Part print with two shaded views. Sizes in mm from the minimum x, y, z corner. Coordinates: 2 decimals unless noted, no trailing zeros. Write each loop counter-clockwise with the first axis right and the second up, starting at its lowest first coordinate (ties: lowest second). Pieces come first, ordered by that corner, then holes. Notation, with made-up numbers: M 78,32.25 L 95,32.25 A25 ccw 95,69.25 Z; hole C -25.5,40.25 d1. An arc over 180 degrees is marked long. One line per question, with ' | ' between items. Start each with the question number.
(1) Wall check: probe 1 along Z at (x, y) = (8, 0.95); probe 2 along X at (y, z) = (0.7, 5.25); probe 3 along Z at (x, y) = (9.25, 0.8). Give the ranges that are in metal, low to high.
(2) Cut at D-D (x = 2). Write the cut outline in (y, z).
(3) Cut at C-C (y = 0.85). Count the separate pieces of the cut face and the enclosed holes in it.
(4) Cut at A-A (z = 1.5). Write the cut outline in (x, y) (1 decimal).
(5) Two-plate mould, pull along X, no slides. Class the marked faces 1, 2 and 3: +X half, -X half, draft (parallel to the pull), parting line (faces both ways), or undercut.
(6) Cut at B-B (x = 10.5). Write the cut outline in (y, z) (1 decimal).
(7) Flat gauge pins, fed straight in: pin 1 Ø1.5 at (x, z) = (2, 5.5) entering from -Y; pin 2 Ø0.5 at (y, z) = (0.5, 4) entering from -X. Where does each tip first touch, or does it go through?
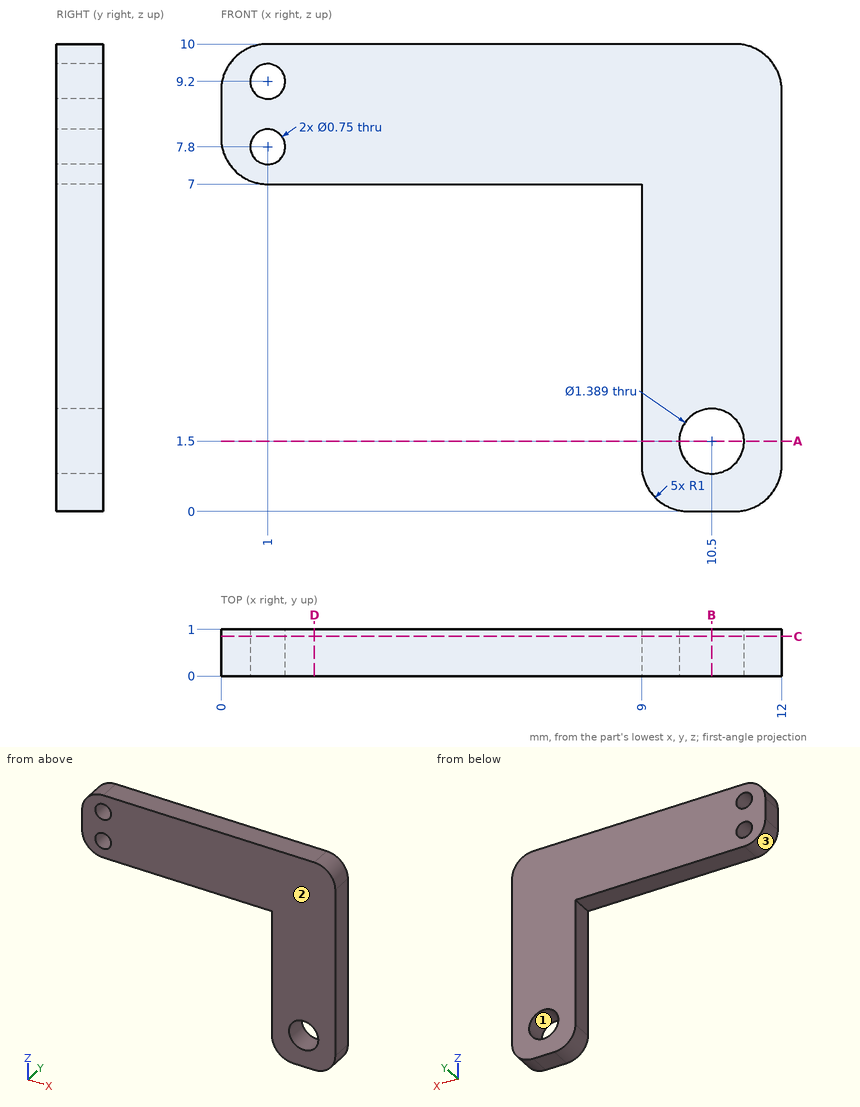
Filled in:
1) probe 1: 7 to 10 | probe 2: 9 to 12 | probe 3: 0.34 to 10
2) outline: M 0,7 L 1,7 L 1,10 L 0,10 Z
3) separate pieces: 1 | enclosed holes: 3
4) outline: M 9,0 L 9.8,0 L 9.8,1 L 9,1 Z; M 11.2,0 L 12,0 L 12,1 L 11.2,1 Z
5) face 1: undercut | face 2: draft | face 3: -X half
6) outline: M 0,0 L 1,0 L 1,0.8 L 0,0.8 Z; M 0,2.2 L 1,2.2 L 1,10 L 0,10 Z
7) pin 1: through | pin 2: x = 9
